Verification items for the finished model (mm, model axes). Round coordinates to 2 decimals unless told otherwise and drop trailing zeros. Write each loop counter-clockwise with the first axis right and the second up, starting at its lowest first coordinate (ties: lowest second). Pieces come first, ordered by that corner, then holes. Notation, with made-up numbers: (76.25, 79) -> (113.25, 79) arc R28 ccw to (113.25, 109) -> close; hole circle Ø4 at (8, 32). An arc over 180 degrees is marked (long way). Use CSV: the item, a comma, the result in double quotes.
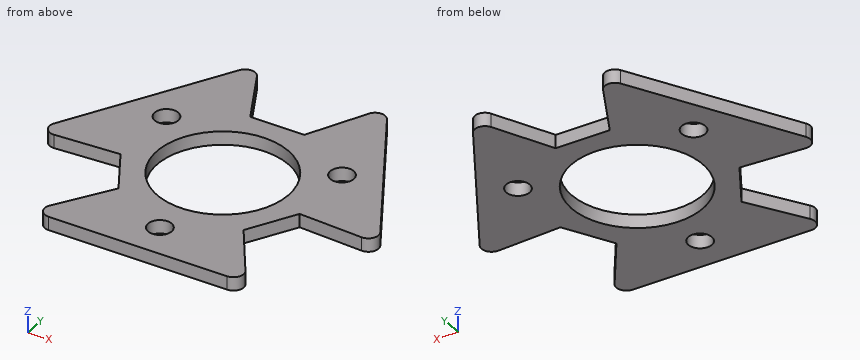
```python
from build123d import *

# Parameters (mm, degrees)
F0_R     = 3.5
F0_R_2   = 19.5
F1_DEPTH = 2
F2_R     = 3


with BuildPart() as f1:
    # F0 (on Top) → F1 (new body, symmetric)
    with BuildSketch(Plane.XY):
        Polygon((-8, 26), (-19.074029, 47.962813), (-51.074029, -7.462813), (-26.51666, -6.071797), (-18.51666, -19.928203), (-32, -40.5), (32, -40.5), (18.51666, -19.928203), (26.51666, -6.071797), (51.074029, -7.462813), (19.074029, 47.962813), (8, 26), align=None)
        with Locations((0, -30.02)):
            Circle(F0_R, mode=Mode.SUBTRACT)
        Circle(F0_R_2, mode=Mode.SUBTRACT)
        with Locations((-25.998083, 15.01)):
            Circle(F0_R, mode=Mode.SUBTRACT)
        with Locations((25.998083, 15.01)):
            Circle(F0_R, mode=Mode.SUBTRACT)
    extrude(amount=F1_DEPTH, both=True)

    # F2
    f2_edges = [f1.edges().sort_by_distance(p)[0] for p in [
        (51.074029, -7.462813, 0),
        (32, -40.5, 0),
        (-19.074029, 47.962813, 0),
        (19.074029, 47.962813, 0),
        (-51.074029, -7.462813, 0),
        (-32, -40.5, 0),
    ]]
    fillet(f2_edges, radius=F2_R)


solid = f1.part
```
Q1. Go/stop test with flat-tipped pins: P1, Ø2, axis at y = -26.5, z = 1.5, coming from the +X side; P2, Ø10, axis at x = 1.5, y = 14.5, coming from the +Z side. Record where each tip stops, or that it passes through.
Filled in:
P1,"x = 23.48"
P2,"z = 2"
Q2. Material ranges on L1, parallel to Y at x = 0, z = -1; L2, parallel to Y at x = 0.5, z = -0.05; L3, parallel to X at y = -3, z = 0.3, recorded low to high.
Filled in:
L1,"-40.5 to -33.52, -26.52 to -19.5, 19.5 to 26"
L2,"-40.5 to -33.48, -26.56 to -19.49, 19.49 to 26"
L3,"-48.47 to -19.27, 19.27 to 48.47"
Q3. Section check D-D (y = 15.01). Record the cut outline in (x, z), plus the area to 3 significant figures.
Filled in:
outline,"(-38.1, -2) -> (-29.5, -2) -> (-29.5, 2) -> (-38.1, 2) -> close; (-22.5, -2) -> (-12.45, -2) -> (-12.45, 2) -> (-22.5, 2) -> close; (12.45, -2) -> (22.5, -2) -> (22.5, 2) -> (12.45, 2) -> close; (29.5, -2) -> (38.1, -2) -> (38.1, 2) -> (29.5, 2) -> close"
area,"149 mm²"
Q4. Section check C-C (y = 0). Record the cut outline in (x, z), plus the area to 3 significant figures.
Filled in:
outline,"(-46.77, -2) -> (-19.5, -2) -> (-19.5, 2) -> (-46.77, 2) -> close; (19.5, -2) -> (46.77, -2) -> (46.77, 2) -> (19.5, 2) -> close"
area,"218 mm²"
Q5. Section check B-B (z = -0.1). Record the cut outline in (x, y).
Filled in:
outline,"(-48.3, -2.65) arc R3 ccw to (-45.53, -7.15) -> (-26.52, -6.07) -> (-18.52, -19.93) -> (-28.96, -35.86) arc R3 ccw to (-26.45, -40.5) -> (26.45, -40.5) arc R3 ccw to (28.96, -35.86) -> (18.52, -19.93) -> (26.52, -6.07) -> (45.53, -7.15) arc R3 ccw to (48.3, -2.65) -> (21.85, 43.15) arc R3 ccw to (16.57, 43) -> (8, 26) -> (-8, 26) -> (-16.57, 43) arc R3 ccw to (-21.85, 43.15) -> close; hole circle Ø7 at (-26, 15.01); hole circle Ø39 at (0, 0); hole circle Ø7 at (0, -30.02); hole circle Ø7 at (26, 15.01)"
Q6. Section check A-A (x = 0). Record the cut outline in (y, z), plus the area to 3 significant figures.
Filled in:
outline,"(-40.5, -2) -> (-33.52, -2) -> (-33.52, 2) -> (-40.5, 2) -> close; (-26.52, -2) -> (-19.5, -2) -> (-19.5, 2) -> (-26.52, 2) -> close; (19.5, -2) -> (26, -2) -> (26, 2) -> (19.5, 2) -> close"
area,"82.0 mm²"
